Can you work these out from the model? Positions are in its coordinate system, mm. Face numbers are marked on the shaded views. A direction names the side the tool comes from. Coordinates: 2 decimals unless noted, no trailing zeros. Order: outer loops, then holes, each group sorted by start corner. A loop starts at its lowest first (then second) coordinate and runs counter-clockwise, first axis right, second up. Notation, with made-up numbers: (23.25, 3) - (74.25, 3) arc R31 cw to (74.25, 28) - close; hole circle Ø10 at (35.25, -38.5). An arc over 180 degrees is marked (long way). Return JSON: item names as keys, results as strings. Group by question number.
1) For pin 1 Ø1 at (x, y) = (11.5, -111.5) entering from +Z, with a flat end and sliding along its axis, tell me the tip position at first contact or that it passes through.
2) Imagine slicing it at B-B (y = -110.5). Write out the boundary of the cut face in (x, z), and give its area (3 significant figures).
3) If we mould it in two halves opening along Y, with no side actions, what happens to the marked faces 1, 2, 3 and 4? For each: pulls with the +Y half, pulls with the -Y half, needs draft (parallel to the pull), parting line crosses it, or undercut.
4) Imagine slicing it at C-C (z = -1.3). Write out the boundary of the cut face in (x, y), and give its area (3 significant figures).
5) Which directions (+Z, -Z, +X, -X, +Y, -Y) give clear straight access to the entire face, cutting with the end or side of a thin tool? Please do the marked faces 5 and 6.
6) Imagine slicing it at A-A (x = 12.25). Write out the boundary of the cut face in (y, z).
7) If I drill on line 1 along Y through (x, z) = (15.25, -1.4); line 2 along X through (y, z) = (-111, -0.55); line 3 along X through (y, z) = (-110.5, -1.25), over which ranges is the centre line in solid material (lowest first)?
8) Imagine slicing it at D-D (x = 19). Write out the boundary of the cut face in (y, z), and give its area (3 significant figures).
```python
from build123d import *

# Parameters (mm, degrees)
SKETCH1_W           = 14.2875
SKETCH1_H           = 14.2875
SKETCH1_W_2         = 12.0015
SKETCH1_H_2         = 12.0015
BOSS_EXTRUDE1_DEPTH = 2.54
SKETCH2_W           = 13.1445
SKETCH2_H           = 13.1445
CUT_EXTRUDE1_DEPTH  = 1.778
FILLET1_R           = 0.508


with BuildPart() as part:
    # Sketch1 → Boss-Extrude1 (new body)
    with BuildSketch(Plane.XY):
        with Locations((12.7, -106.3625)):
            Rectangle(SKETCH1_W, SKETCH1_H)
        with Locations((12.7, -106.3625)):
            Rectangle(SKETCH1_W_2, SKETCH1_H_2, mode=Mode.SUBTRACT)
    extrude(amount=-BOSS_EXTRUDE1_DEPTH)

    # Sketch2 → Cut-Extrude1 (cut)
    with BuildSketch(Plane(origin=(0, 0, -2.54), x_dir=(-1, 0, 0), z_dir=(0, 0, -1))):
        with Locations((-12.7, -106.3625)):
            Rectangle(SKETCH2_W, SKETCH2_H)
    extrude(amount=-CUT_EXTRUDE1_DEPTH, mode=Mode.SUBTRACT)

    # Fillet1
    fillet1_edges = [part.edges().sort_by_distance(p)[0] for p in [
        (5.55625, -106.3625, 0),
        (12.7, -99.21875, 0),
        (19.84375, -106.3625, 0),
        (12.7, -113.50625, 0),
        (5.55625, -113.50625, -1.27),
        (5.55625, -99.21875, -1.27),
        (19.84375, -99.21875, -1.27),
        (19.84375, -113.50625, -1.27),
    ]]
    fillet(fillet1_edges, radius=FILLET1_R)


solid = part.part
```
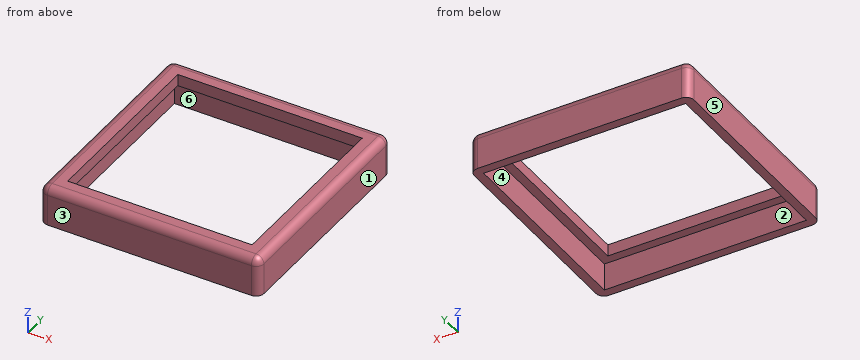
Calculated:
{
 "1": {"pin 1": "through"},
 "2": {"outline": "(5.56, -2.54) - (6.13, -2.54) - (6.13, -0.76) - (6.7, -0.76) - (6.7, 0) - (6.06, 0) arc R0.51 ccw to (5.56, -0.51) - close; (18.7, -0.76) - (19.27, -0.76) - (19.27, -2.54) - (19.84, -2.54) - (19.84, -0.51) arc R0.51 ccw to (19.34, 0) - (18.7, 0) - close", "area": "3.66 mm2"},
 "3": {"face 1": "needs draft", "face 2": "undercut", "face 3": "pulls with the -Y half", "face 4": "undercut"},
 "4": {"outline": "(5.56, -113) arc R0.51 ccw to (6.06, -113.51) - (19.34, -113.51) arc R0.51 ccw to (19.84, -113) - (19.84, -99.73) arc R0.51 ccw to (19.34, -99.22) - (6.06, -99.22) arc R0.51 ccw to (5.56, -99.73) - close; hole (6.13, -112.93) - (19.27, -112.93) - (19.27, -99.79) - (6.13, -99.79) - close", "area": "31.1 mm2"},
 "5": {"face 5": "+Z, -Z, -X, +Y, -Y", "face 6": "-Z"},
 "6": {"outline": "(-113.51, -2.54) - (-112.93, -2.54) - (-112.93, -0.76) - (-112.36, -0.76) - (-112.36, 0) - (-113, 0) arc R0.51 ccw to (-113.51, -0.51) - close; (-100.36, -0.76) - (-99.79, -0.76) - (-99.79, -2.54) - (-99.22, -2.54) - (-99.22, -0.51) arc R0.51 ccw to (-99.73, 0) - (-100.36, 0) - close"},
 "7": {"line 1": "-113.51 to -112.93, -99.79 to -99.22", "line 2": "5.56 to 6.7, 18.7 to 19.84", "line 3": "5.56 to 6.13, 19.27 to 19.84"},
 "8": {"outline": "(-113.51, -2.54) - (-112.93, -2.54) - (-112.93, -0.76) - (-99.79, -0.76) - (-99.79, -2.54) - (-99.22, -2.54) - (-99.22, -0.51) arc R0.51 ccw to (-99.73, 0) - (-113, 0) arc R0.51 ccw to (-113.51, -0.51) - close", "area": "12.8 mm2"}
}
